```python
from build123d import *

# Parameters (mm, degrees)
BOSS_EXTRUDE1_DEPTH = 3
CUT_EXTRUDE1_DEPTH  = 1.5
BOSS_EXTRUDE2_DEPTH = 1.5
BOSS_EXTRUDE3_DEPTH = 4.5
BOSS_EXTRUDE4_DEPTH = 4.5


with BuildPart() as part:
    # Sketch1 → Boss-Extrude1 (new body)
    with BuildSketch(Plane(origin=(0, 0, 0), x_dir=(1, 0, 0), z_dir=(0, 1, 0))):
        Polygon((-7.5, 3.5), (-7.5, -3.5), (7.5, -3), (7.5, 3), align=None)
    extrude(amount=BOSS_EXTRUDE1_DEPTH)

    # Sketch2 → Cut-Extrude1 (cut)
    with BuildSketch(Plane.XZ):
        with BuildLine():
            Line((-7.5, 2.375), (-7.5, -2.375))
            Line((-7.5, -2.375), (-0.032313986, -2.025))
            ThreePointArc((-0.032313986, -2.025), (1.9, 0), (-0.032313986, 2.025))
            Line((-0.032313986, 2.025), (-7.5, 2.375))
        make_face()
    extrude(amount=-CUT_EXTRUDE1_DEPTH, mode=Mode.SUBTRACT)

    # Sketch4 → Boss-Extrude2 (add)
    with BuildSketch(Plane.XZ):
        Polygon((-7.5, -3.5), (7.5, -3), (7.5, 3), (-7.5, 3.5), align=None)
    extrude(amount=BOSS_EXTRUDE2_DEPTH)

    # Sketch6 → Boss-Extrude3 (add)
    with BuildSketch(Plane(origin=(0, 3, 0), x_dir=(1, 0, 0), z_dir=(0, 1, 0))):
        with BuildLine():
            Line((7.5, 7.5), (7.5, -7.5))
            ThreePointArc((7.5, -7.5), (11.5, 0), (7.5, 7.5))
        make_face()
    extrude(amount=-BOSS_EXTRUDE3_DEPTH)

    # Sketch7 → Boss-Extrude4 (add)
    with BuildSketch(Plane.XZ.offset(1.5)):
        Polygon((7.5, 7.5), (0, 3.25), (7.5, 3), align=None)
    boss_extrude4 = extrude(amount=-BOSS_EXTRUDE4_DEPTH)

    # Mirror1: Boss-Extrude4 across plane
    add(boss_extrude4.mirror(Plane.XY))


solid = part.part
```
Can you work these out from the model? Positions are in its coordinate system, mm. A direction names the side the tool comes from. Coordinates: 2 decimals unless noted, no trailing zeros. Loops run counter-clockwise (first coordinate to the right, second up) from the corner with the lowest first, then second, coordinate; pieces in that order, holes last.
Item 1: If we mould it in two halves opening along Z, with no side actions, what happens to faces 1 (the face through (-3, 1.5, 0)), 2 (the face through (4, 3, 0)), 3 (the face through (3.802, 0.719, -5.405))? For each: released by +Z, released by -Z, zero draft, split by the parting line, or undercut.
Answers below:
face 1: undercut
face 2: zero draft
face 3: released by -Z
Item 2: I'm going to push flat-ended pins straight in: pin 1 (2 mm diameter, centred on x = 8, y = -0.5, fed in from -Z); pin 2 (2 mm diameter, centred on x = 6, y = -0.5, fed in from -Z); pin 3 (1.5 mm diameter, centred on y = 1.5, z = 5.5, fed in from -X). Where does each tip first touch, or does it pass through?
Answers below:
pin 1: stops at z = -7.5
pin 2: stops at z = -7.22
pin 3: stops at x = 2.65
Item 3: Please list where these lines run through material, in increasing order: L1, parallel to Z at x = -5.5, y = 1.05; L2, parallel to X at y = 0.05, z = 0.75; L3, parallel to X at y = -1.1, z = 2.75.
Answers below:
L1: z = -3.43 to -2.28, 2.28 to 3.43
L2: x = 1.76 to 11.47
L3: x = -7.5 to 11.07
Item 4: Suppose I cut it at C-C (z = -1.75). Please give me the cut outline in (x, y).
Answers below:
outline: (-7.5, -1.5) - (11.33, -1.5) - (11.33, 3) - (-7.5, 3) - (-7.5, 1.5) - (0.9, 1.5) - (0.9, 0) - (-7.5, 0) - close
Item 5: Suppose I cut it at D-D (y = -1.2). Please give me the cut outline in (x, z), then the cut area to 3 significant figures.
Answers below:
outline: (-7.5, -3.5) - (0, -3.25) - (7.5, -7.5) arc R9.03 ccw to (7.5, 7.5) - (0, 3.25) - (-7.5, 3.5) - close
area: 173 mm2
Item 6: Which directions (+Z, -Z, +X, -X, +Y, -Y) give clear straight access to the entire face, cutting with the end or side of a thin tool? Please do faces 4 (the face through (4, -1.5, 0)), 5 (the face through (-3.714, 0.74, 2.198)).
Answers below:
face 4: +Z, -Z, +X, -X, -Y
face 5: -X
Item 7: Suppose I cut it at B-B (z = 0). Please give me the cut outline in (x, y), then the cut area to 3 significant figures.
Answers below:
outline: (-7.5, -1.5) - (11.5, -1.5) - (11.5, 3) - (-7.5, 3) - (-7.5, 1.5) - (1.9, 1.5) - (1.9, 0) - (-7.5, 0) - close
area: 71.4 mm2
